Geometry check sheet. Reference: the model listing, model coordinates, mm. A direction names the side the tool comes from. Round coordinates to 2 decimals unless told otherwise and drop trailing zeros. Order: outer loops, then holes, each group sorted by start corner. A loop starts at its lowest first (then second) coordinate and runs counter-clockwise, first axis right, second up.
(1) Set-up check for faces 1 (the face through (11.923, 7.395, 3.755)), 2 (the face through (-2.76, -4.76, -12.44)): record each of +Z, -Z, +X, -X, +Y, -Y from which the full face is reachable in a straight line by a thin tool's end or side.
(2) Sectioned sample at D-D (y = 10.5). Record the boundary of the cut face in (x, z).
(3) Sectioned sample at C-C (y = 6.5). Record the boundary of the cut face in (x, z), plus the area to 3 significant figures.
(4) Go/stop test with flat-tipped pins: pin 1 (12 mm diameter, centred on x = -7, y = 8, fed in from +Z); pin 2 (3 mm diameter, centred on x = 7, z = -12.5, fed in from +Y); pin 3 (6 mm diameter, centred on y = 4, z = -1.5, fed in from -X). Record where each tip stops, or that it passes through.
(5) Material ranges on line 1 along Z through (x, y) = (0, 3.45); line 2 along Z through (x, y) = (5.5, -2.75); line 3 along X through (y, z) = (2.25, -1.5), recorded low to high.
from build123d import *

# Parameters (mm, degrees)
F0_R     = 17.5
F0_R_2   = 12.5
F0_R_3   = 10
F1_DEPTH = 5
F2_DEPTH = 15
F4_SIZE  = 4.99999


# Not quite as in the source:
# - a fillet or chamfer that OpenCascade refuses, or shapes differently, is made with other operations: its cross-section is extruded or revolved along the edge and cut away or added
# - a fillet or chamfer is up to 0.001 mm smaller than in the source, because OpenCascade refuses the exact size


with BuildPart() as f1:
    # F0 (on Front) → F1 (new body)
    with BuildSketch(Plane.XZ):
        Circle(F0_R)
        Circle(F0_R_2, mode=Mode.SUBTRACT)
        Circle(F0_R_2)
        Circle(F0_R_3, mode=Mode.SUBTRACT)
    extrude(amount=F1_DEPTH)

    # F0 (on Front) → F2 (join)
    with BuildSketch(Plane.XZ):
        Circle(F0_R_2)
        Circle(F0_R_3, mode=Mode.SUBTRACT)
    extrude(amount=-F2_DEPTH)

    # F3: fillet of radius 22 on 1 edges, made by hand

    # F3_s1 → F3_t2 (revolve, cut)
    with BuildSketch(Plane.XY):
        with BuildLine():
            ThreePointArc((10, 4.8142256063), (10.6341393808, 10.0582698471), (12.5, 15))
            Line((12.5, 15), (10, 15))
            Line((10, 15), (10, 4.8142256063))
        make_face()
    revolve(axis=Axis((0, 15, 0), (0, -1, 0)), mode=Mode.SUBTRACT)

    # F4 (size 5 in the source; OpenCascade refuses exactly that, so slightly less here)
    f4_edges = [f1.edges().sort_by_distance(p)[0] for p in [
        (-17.5, -5, 0),
    ]]
    chamfer(f4_edges, length=F4_SIZE)


solid = f1.part
Answer below:
1. face 1: +Y
1. face 2: -Y
2. outline: circle Ø25 at (0, 0); hole circle Ø21.49 at (0, 0)
3. outline: circle Ø25 at (0, 0); hole circle Ø20.13 at (0, 0)
3. area: 173 mm2
4. pin 1: stops at z = 12.46
4. pin 2: stops at y = 0
4. pin 3: stops at x = -12.5
5. line 1: z = -12.5 to -10, 10 to 12.5
5. line 2: z = -13.69 to -8.35, 8.35 to 13.69
5. line 3: x = -12.41 to -9.89, 9.89 to 12.41
